Could you check a few things on this drawing? It's one solid part, dimensions in mm from its lowest x, y, z. Give positions to 0.01 mm unless a question says otherwise; leave off trailing zeros. Loops run counter-clockwise (first coordinate to the right, second up) from the corner with the lowest first, then second, coordinate; pieces in that order, holes last.
Q1. Suppose I cut it at B-B (z = 25). List the corners of the cut face in (x, y) for me, and give its area (3 significant figures).
Q2. Suppose I cut it at D-D (x = 5). List the corners of the cut face in (y, z) for me, and give its area (3 significant figures).
Q3. I'm going to push a flat-ended pin straight in: P1, Ø12, axis at y = 60, z = 95, coming from the -X side. Where does the tip first touch, or does it pass through?
Q4. I need wall thicknesses on probe 1 along Y at (x, z) = (3, 25); probe 2 along Z at (x, y) = (1.5, 27.5); probe 3 along Z at (x, y) = (5.25, 60). Which ranges of each line are inside material? Lowest first, please.
Q5. Suppose I cut it at A-A (z = 95). List the corners of the cut face in (x, y) for me, and give its area (3 significant figures).
Q6. Suppose I cut it at C-C (y = 60). List the corners of the cut face in (x, z) for me, and give its area (3 significant figures).
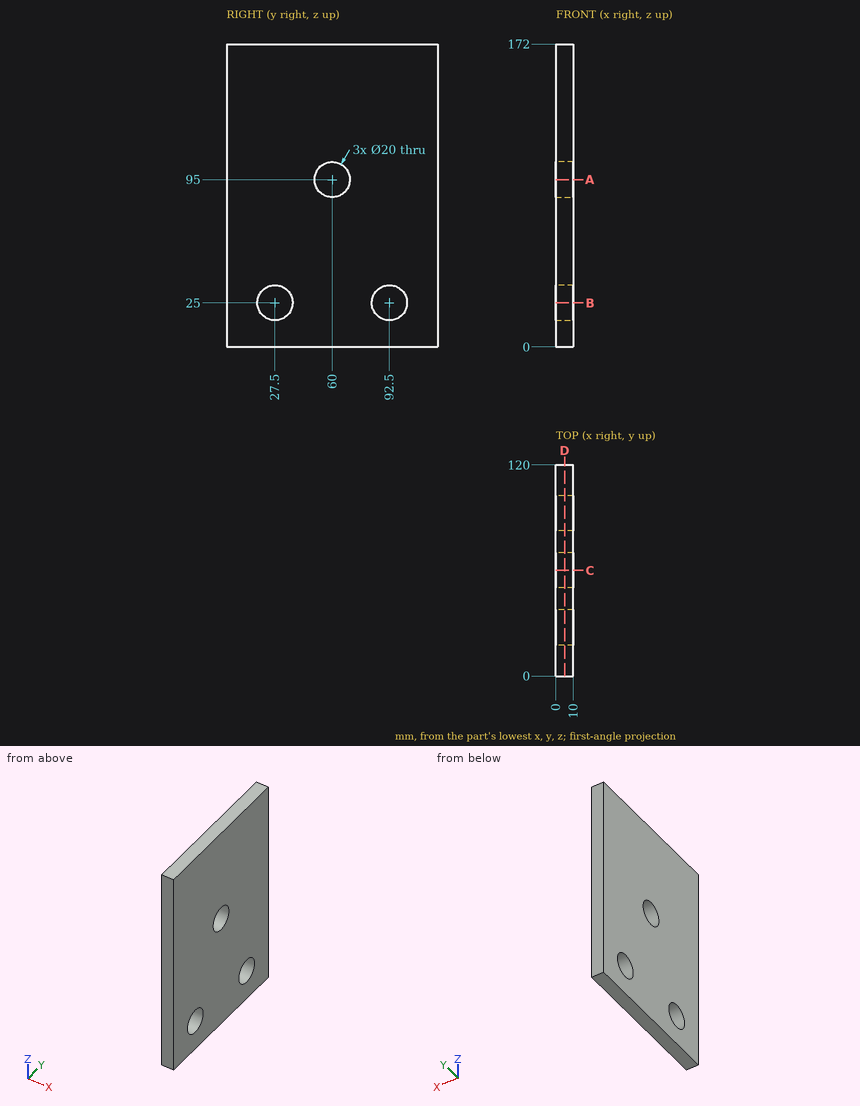
Solutions:
1. outline: (0, 0) - (10, 0) - (10, 17.5) - (0, 17.5) - close; (0, 37.5) - (10, 37.5) - (10, 82.5) - (0, 82.5) - close; (0, 102.5) - (10, 102.5) - (10, 120) - (0, 120) - close
1. area: 800 mm2
2. outline: (0, 0) - (120, 0) - (120, 172) - (0, 172) - close; hole circle Ø20 at (27.5, 25); hole circle Ø20 at (60, 95); hole circle Ø20 at (92.5, 25)
2. area: 19,700 mm2
3. P1: passes through
4. probe 1: y = 0 to 17.5, 37.5 to 82.5, 102.5 to 120
4. probe 2: z = 0 to 15, 35 to 172
4. probe 3: z = 0 to 85, 105 to 172
5. outline: (0, 0) - (10, 0) - (10, 50) - (0, 50) - close; (0, 70) - (10, 70) - (10, 120) - (0, 120) - close
5. area: 1,000 mm2
6. outline: (0, 0) - (10, 0) - (10, 85) - (0, 85) - close; (0, 105) - (10, 105) - (10, 172) - (0, 172) - close
6. area: 1,520 mm2
